The figure shows three views and two pictorial views of one solid part (mm, origin at its lowest corner). Answer the questions. A direction names the side the tool comes from. Coordinates: 2 decimals unless noted, no trailing zeros. Loops run counter-clockwise (first coordinate to the right, second up) from the corner with the lowest first, then second, coordinate; pieces in that order, holes last. Notation, with made-up numbers: (37.25, 82.5) - (63.25, 82.5) arc R14 ccw to (63.25, 103.5) - close; hole circle Ø6 at (15, 69). An arc over 180 degrees is marked (long way). One line per question, with ' | ' between items.
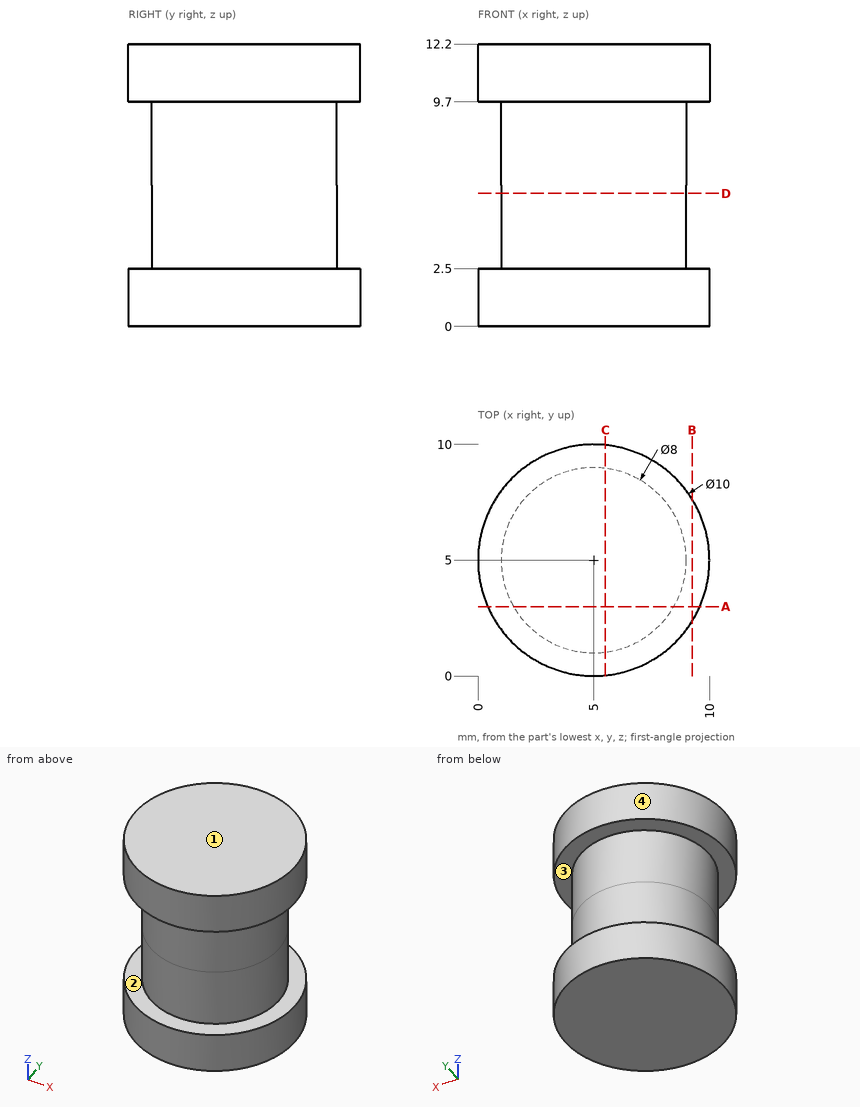
Item 1: Each of these flat-tipped pins is pushed along its axis until it touches: pin 1 Ø4 at (x, y) = (5, 3) entering from -Z; pin 2 Ø4 at (y, z) = (8, 9) entering from -X; pin 3 Ø3 at (y, z) = (7, 2.5) entering from -X; pin 4 Ø3 at (x, z) = (7.5, 11) entering from +Y. Where does it stop, or does it pass through?
Taken from the geometry:
pin 1: stops at z = 0 | pin 2: stops at x = 0.13 | pin 3: stops at x = 0.03 | pin 4: stops at y = 9.9
Item 2: Find section B-B, the plane x = 9.25. Write down the section's boundary in (y, z).
Taken from the geometry:
outline: (2.37, 0) - (7.63, 0) - (7.63, 2.5) - (2.37, 2.5) - close; (2.37, 9.7) - (7.63, 9.7) - (7.63, 12.2) - (2.37, 12.2) - close
Item 3: Find the intervals of material crossed by line 1 (Z direction, x = 9, y = 6); line 2 (Y direction, x = 7.25, z = 4.75); line 3 (X direction, y = 4, z = 4), in increasing order. Write a range as [from, to].
Taken from the geometry:
line 1: z = [0, 2.5], [9.7, 12.2] | line 2: y = [1.69, 8.31] | line 3: x = [1.13, 8.87]
Item 4: Find section D-D, the plane z = 5.75. Write down the section's boundary in (x, y).
Taken from the geometry:
outline: circle Ø8 at (5, 5)
Item 5: Find section A-A, the plane y = 3. Write down the section's boundary in (x, z).
Taken from the geometry:
outline: (0.42, 0) - (9.58, 0) - (9.58, 2.5) - (8.46, 2.5) - (8.46, 9.7) - (9.58, 9.7) - (9.58, 12.2) - (0.42, 12.2) - (0.42, 9.7) - (1.54, 9.7) - (1.54, 2.5) - (0.42, 2.5) - close
Item 6: Which of the six approach directions +Z, -Z, +X, -X, +Y, -Y give full straight-line access (tool end or side, diameter ignored) to the marked faces 1 and 2?
Taken from the geometry:
face 1: +Z, +X, -X, +Y, -Y | face 2: none
Item 7: The mould has two halves that part along Y. Classify the marked faces 3 and 4: pulls with the +Y half, pulls with the -Y half, needs draft (parallel to the pull), parting line crosses it, or undercut.
Taken from the geometry:
face 3: needs draft | face 4: parting line crosses it
Item 8: Find section C-C, the plane x = 5.5. Write down the section's boundary in (y, z).
Taken from the geometry:
outline: (0.03, 0) - (9.97, 0) - (9.97, 2.5) - (8.97, 2.5) - (8.97, 9.7) - (9.97, 9.7) - (9.97, 12.2) - (0.03, 12.2) - (0.03, 9.7) - (1.03, 9.7) - (1.03, 2.5) - (0.03, 2.5) - close
